For this review, take the finished solid that the model builds, in its own axes (mm). A direction names the side the tool comes from. Give positions to 0.01 mm unless a question says otherwise; leave off trailing zeros. Loops run counter-clockwise (first coordinate to the right, second up) from the corner with the lowest first, then second, coordinate; pieces in that order, holes last.
```python
from build123d import *

# Parameters (mm, degrees)
F1_DEPTH       = 40
F3_W           = 30
F3_H           = 28
F3_H_2         = 45
F4_DEPTH       = 14.1
F6_D           = 5.25
F6_DEPTH       = 5
F6_CBORE_D     = 9.75
F6_CBORE_DEPTH = 1.6
F6_TIP         = 1.5772591249
F7_D           = 2.5
F7_DEPTH       = 10
F7_TIP         = 0.7510757738


# Not quite as in the source:
# - a feature names something its author has since deleted; it is built from what else it names


with BuildPart() as f1:
    # F0 (on Right) → F1 (new body)
    with BuildSketch(Plane.YZ):
        Polygon((0, 0), (-78, 0), (-78, 16.5), (-83, 16.5), (-83, -8.5), (0, -8.5), align=None)
        Polygon((-78, 16.5), (-78, 0), (0, 0), (-50, 16.5), align=None)
    extrude(amount=F1_DEPTH)

    # F3 (on face) → F4 (cut)
    with BuildSketch(Plane.XY.offset(16.5)):
        with Locations((20, -64)):
            Rectangle(F3_W, F3_H)
        with Locations((20, -27.5)):
            Rectangle(F3_W, F3_H_2)
    extrude(amount=-F4_DEPTH, mode=Mode.SUBTRACT)

    # F6
    with Locations(Plane(origin=(0, -78, 0), x_dir=(-1, 0, 0), z_dir=(0, 1, 0))):
        with Locations((-30, 7.5), (-10, 7.5)):
            CounterBoreHole(F6_D / 2, F6_CBORE_D / 2, F6_CBORE_DEPTH, depth=F6_DEPTH)
            with Locations((0, 0, -(F6_DEPTH + F6_TIP / 2))):  # 118° drill point
                Cone(0, F6_D / 2, F6_TIP, mode=Mode.SUBTRACT)

    # F7
    with Locations(Plane(origin=(0, 0, -8.5), x_dir=(1, 0, 0), z_dir=(0, 0, -1))):
        with Locations((24, 30), (24, 19), (32, 19), (24, 8)):
            Hole(F7_D / 2, depth=F7_DEPTH)
            with Locations((0, 0, -(F7_DEPTH + F7_TIP / 2))):  # 118° drill point
                Cone(0, F7_D / 2, F7_TIP, mode=Mode.SUBTRACT)


solid = f1.part
```
Item 1: The part is to be moulded in two halves that separate along Z. For faces 1 (the cylindrical face through (7.378, -81.324, 7.615)), 2 (the conical face through (32.21, -19.07, 2.12)), 3 (the flat face through (40, -51, 1)), say which applies: released by +Z, released by -Z, zero draft, split by the parting line, or undercut.
Answer:
face 1: undercut
face 2: released by -Z
face 3: zero draft
Item 2: Clearance check with flat-ended pins moving along their axes: pin 1 Ø5 at (x, y) = (26, -22.5) entering from +Z; pin 2 Ø2 at (x, y) = (24, -30) entering from -Z; pin 3 Ø2 at (x, y) = (5.5, -36.5) entering from +Z. State where each tip first meets the part, or that it passes through.
Answer:
pin 1: stops at z = 2.4
pin 2: stops at z = 1.65
pin 3: stops at z = 12.33
Item 3: Take a section at D-D on x = 20. Give the boundary of the cut face in (y, z), and give its area (3 significant figures).
Answer:
outline: (-83, -8.5) - (0, -8.5) - (0, 0) - (-7.27, 2.4) - (-78, 2.4) - (-78, 16.5) - (-83, 16.5) - close
area: 966 mm2
Item 4: Take a section at B-B on y = -48. Give the boundary of the cut face in (x, z).
Answer:
outline: (0, -8.5) - (40, -8.5) - (40, 15.84) - (35, 15.84) - (35, 2.4) - (5, 2.4) - (5, 15.84) - (0, 15.84) - close
Item 5: Take a section at C-C on z = 7.5. Give the boundary of the cut face in (x, y) (3 decimals).
Answer:
outline: (0, -83) - (7.375, -83) - (7.375, -79.6) - (5.125, -79.6) - (5.125, -78) - (5, -78) - (5, -22.727) - (0, -22.727) - close; (12.625, -83) - (27.375, -83) - (27.375, -79.6) - (25.125, -79.6) - (25.125, -78) - (14.875, -78) - (14.875, -79.6) - (12.625, -79.6) - close; (32.625, -83) - (40, -83) - (40, -22.727) - (35, -22.727) - (35, -78) - (34.875, -78) - (34.875, -79.6) - (32.625, -79.6) - close
Item 6: Take a section at A-A on x = 10. Give the boundary of the cut face in (y, z) (3 decimals), and give its area (3 significant figures).
Answer:
outline: (-83, -8.5) - (0, -8.5) - (0, 0) - (-7.273, 2.4) - (-78, 2.4) - (-78, 2.625) - (-79.6, 2.625) - (-79.6, 4.875) - (-83, 4.875) - close; (-83, 10.125) - (-79.6, 10.125) - (-79.6, 12.375) - (-78, 12.375) - (-78, 16.5) - (-83, 16.5) - close
area: 933 mm2
Item 7: Tool access review of faces 4 (the cylindrical face through (33.869, -78.789, 4.534)), 5 (the cylindrical face through (30.845, -18.521, -3.43)), 6 (the flat face through (35, -51, 8)): name each direction out of +Z, -Z, +X, -X, +Y, -Y from which nothing blocks a thin tool from reaching the whole face with its end or side.
Answer:
face 4: +Y
face 5: -Z
face 6: +Z, +Y
Item 8: For L1, parallel to X at y = -19, z = -6.5; L2, parallel to X at y = -81.25, z = 7.5 (3 decimals); L3, parallel to Y at x = 24, z = -5, list the stretches that pass through material, from the lowest coordinate up.
Answer:
L1: x = 0 to 22.75, 25.25 to 30.75, 33.25 to 40
L2: x = 0 to 7.375, 12.625 to 27.375, 32.625 to 40
L3: y = -83 to -31.25, -28.75 to -20.25, -17.75 to -9.25, -6.75 to 0
